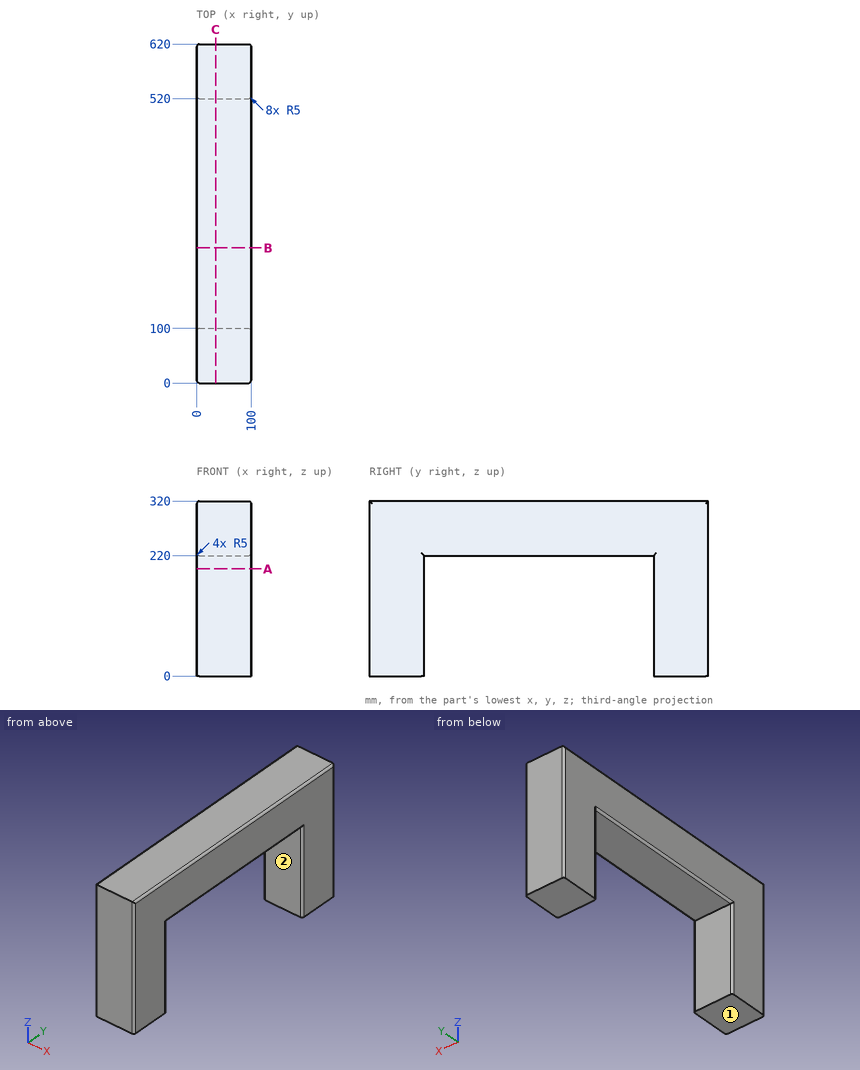
Part print with two shaded views. Sizes in mm from the minimum x, y, z corner. A direction names the side the tool comes from. Coordinates: 2 decimals unless noted, no trailing zeros. Write each loop counter-clockwise with the first axis right and the second up, starting at its lowest first coordinate (ties: lowest second). Pieces come first, ordered by that corner, then holes. Notation, with made-up numbers: (-32.75, 36) -> (-12.75, 36) arc R35 cw to (-12.75, 70) -> close; hole circle Ø7 at (-13, -0.5). An arc over 180 degrees is marked (long way). Return JSON: item names as keys, results as strings. Group by question number.
Q1. Cut at A-A, the plane z = 196. Give the cut face in (x, y), then the cut area to 3 significant figures.
Q2. Which spindle directions (+Z, -Z, +X, -X, +Y, -Y) get a long thin tool onto all of the face, cutting with end or side? Do the marked faces 1 and 2. Say none if no direction does.
Q3. Cut at C-C, the plane x = 34.5. Give the cut face in (y, z).
Q4. Flat gauge pins, fed straight in: pin 1 (3 mm diameter, centred on y = 466, z = 220.5, fed in from +X); pin 2 (1.5 mm diameter, centred on x = 31.5, y = 120.5, fed in from -Z). Where does each tip first touch, or does it go through?
Q5. Drill centre lines: line 1 (Y direction, x = 94, z = 96); line 2 (Z direction, x = 15.5, y = 351.5). Where is each one in solid material? Low to high.
Q6. Cut at B-B, the plane y = 247. Give the cut face in (x, z), then the cut area to 3 significant figures.
Returned:
{
 "1": {"outline": "(0, 5) arc R5 ccw to (5, 0) -> (95, 0) arc R5 ccw to (100, 5) -> (100, 95) arc R5 ccw to (95, 100) -> (5, 100) arc R5 ccw to (0, 95) -> close; (0, 525) arc R5 ccw to (5, 520) -> (95, 520) arc R5 ccw to (100, 525) -> (100, 615) arc R5 ccw to (95, 620) -> (5, 620) arc R5 ccw to (0, 615) -> close", "area": "20,000 mm2"},
 "2": {"face 1": "-Z, +X, -X, +Y, -Y", "face 2": "-Z, +X, -X"},
 "3": {"outline": "(0, 0) -> (100, 0) -> (100, 220) -> (520, 220) -> (520, 0) -> (620, 0) -> (620, 320) -> (0, 320) -> close"},
 "4": {"pin 1": "stops at x = 99", "pin 2": "stops at z = 220"},
 "5": {"line 1": "y = 0 to 100, 520 to 620", "line 2": "z = 220 to 320"},
 "6": {"outline": "(0, 225) arc R5 ccw to (5, 220) -> (95, 220) arc R5 ccw to (100, 225) -> (100, 315) arc R5 ccw to (95, 320) -> (5, 320) arc R5 ccw to (0, 315) -> close", "area": "9,980 mm2"}
}
